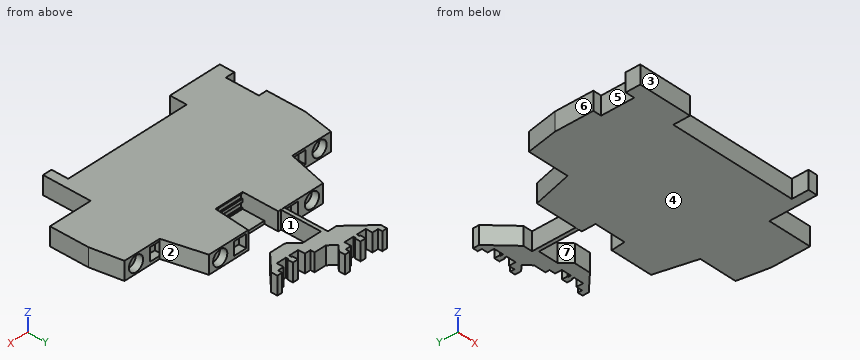
Autodesk Inventor part; units mm, degrees
ref_plane "1_1001_XY" through (7.05, 53.6, 2.5) normal (0, 1, 0) x (-1, 0, 0)
ref_plane "1_1001_YZ" through (7.05, 53.6, 2.5) normal (-1, 0, 0) x (0, 0, 1)
ref_plane "1_1001_ZX" through (7.05, 53.6, 2.5) normal (0, 0, 1) x (0, 1, 0)
sketch "Sketch_1" plane through (0, 0, 0) normal (0, 0, 1) x (1, 0, 0)
  line L0 (-32.2, -0.6) -> (-32.2, -4.6)
  line L1 (-32.2, -4.6) -> (-17.5, -4.6)
  line L2 (-17.5, -4.6) -> (-17.5, 0)
  line L3 (-17.5, 0) -> (17.5, 0)
  line L4 (17.5, 0) -> (17.5, -4.6)
  line L5 (17.5, -4.6) -> (20, -4.6)
  line L6 (20, -4.6) -> (20, 8.5)
  line L7 (20, 8.5) -> (32, 8.5)
  line L8 (32, 8.5) -> (32, 19.1)
  line L9 (32, 19.1) -> (30.5012, 27.6)
  line L10 (30.5012, 27.6) -> (-30.5012, 27.6)
  line L11 (-30.5012, 27.6) -> (-32, 19.1)
  line L12 (-32, 19.1) -> (-32, 8.5)
  line L13 (-32, 8.5) -> (-29.7, 8.5)
  line L14 (-29.7, 8.5) -> (-29.7, -0.6)
  line L15 (-29.7, -0.6) -> (-32.2, -0.6)
extrude "Extrusion1" add sketch "Sketch_1" along normal blind 5
sketch "Sketch_2" plane through (0, 0, 0) normal (0, 0, 1) x (1, 0, 0)
  line L0 (-19.1, 27.6) -> (-18.2, 27.6)
  line L1 (-18.2, 27.6) -> (-18.2, 15.1)
  line L2 (-18.2, 15.1) -> (19.2, 15.1)
  line L3 (19.2, 15.1) -> (19.2, 27.6)
  line L4 (19.2, 27.6) -> (20.1, 27.6)
  line L5 (20.1, 27.6) -> (17.3574, 38.6)
  line L6 (17.3574, 38.6) -> (5.7574, 38.6)
  line L7 (5.7574, 38.6) -> (4.9, 28.8)
  line L8 (4.9, 28.8) -> (-3.1, 28.8)
  line L9 (-3.1, 28.8) -> (-3.1, 38.6)
  line L10 (-3.1, 38.6) -> (-16.3574, 38.6)
  line L11 (-16.3574, 38.6) -> (-19.1, 27.6)
extrude "Extrusion2" add sketch "Sketch_2" along normal blind 5
sketch "Skizze_3" plane through (0, 0, 0) normal (0, 0, 1) x (1, 0, 0)
  line L0 (-3.1, 34.8) -> (-3.1, 28.8)
  line L1 (-3.1, 28.8) -> (5.9, 28.8)
  line L2 (5.9, 28.8) -> (5.9, 34.8)
  line L3 (5.9, 34.8) -> (-3.1, 34.8)
extrude "Extrusion3" add sketch "Skizze_3" along normal blind 0.8
sketch "Sketch_3" plane through (0.5, 0, 0) normal (1, 0, 0) x (0, 0, -1)
  line L0 (-4.7, 28.4) -> (-3.3, 28.4)
  line L1 (-3.3, 28.4) -> (-3.3, 28.8)
  line L2 (-3.3, 28.8) -> (-2.5, 28.8)
  line L3 (-2.5, 28.8) -> (-2.5, 28.4)
  line L4 (-2.5, 28.4) -> (-1.1, 28.4)
  line L5 (-1.1, 28.4) -> (-1.1, 29.8)
  line L6 (-1.1, 29.8) -> (-4.7, 29.8)
  line L7 (-4.7, 29.8) -> (-4.7, 28.4)
extrude "Extrusion4" cut sketch "Sketch_3" along normal mid plane 7.2
sketch "Sketch_4" plane through (0, 0, 2.5) normal (0, 0, 1) x (1, 0, 0)
  line L0 (27.1, 25.6) -> (27.1, 27.6)
  line L1 (27.1, 27.6) -> (29.2, 27.6)
  line L2 (29.2, 27.6) -> (29.2, 25.6)
  line L3 (29.2, 25.6) -> (27.1, 25.6)
  line L4 (27.1, 25.6) -> (27.1, 27.6)
revolve "Revolution1" cut sketch "Sketch_4" angle 360 about axis through (27.1, 25.6, 2.5) along (0, -1, 0)
sketch "Sketch_5" plane through (0, 0, 2.5) normal (0, 0, 1) x (1, 0, 0)
  line L0 (-27.1, 25.6) -> (-27.1, 27.6)
  line L1 (-27.1, 27.6) -> (-25, 27.6)
  line L2 (-25, 27.6) -> (-25, 25.6)
  line L3 (-25, 25.6) -> (-27.1, 25.6)
  line L4 (-27.1, 25.6) -> (-27.1, 27.6)
revolve "Revolution2" cut sketch "Sketch_5" angle 360 about axis through (-27.1, 25.6, 2.5) along (0, -1, 0)
sketch "Sketch_6" plane through (0, 0, 2.5) normal (0, 0, 1) x (1, 0, 0)
  line L0 (14.05, 36.6) -> (14.05, 38.6)
  line L1 (14.05, 38.6) -> (16.15, 38.6)
  line L2 (16.15, 38.6) -> (16.15, 36.6)
  line L3 (16.15, 36.6) -> (14.05, 36.6)
  line L4 (14.05, 36.6) -> (14.05, 38.6)
revolve "Revolution3" cut sketch "Sketch_6" angle 360 about axis through (14.05, 36.6, 2.5) along (0, -1, 0)
sketch "Sketch_7" plane through (0, 0, 2.5) normal (0, 0, 1) x (1, 0, 0)
  line L0 (-13.05, 36.6) -> (-13.05, 38.6)
  line L1 (-13.05, 38.6) -> (-10.95, 38.6)
  line L2 (-10.95, 38.6) -> (-10.95, 36.6)
  line L3 (-10.95, 36.6) -> (-13.05, 36.6)
  line L4 (-13.05, 36.6) -> (-13.05, 38.6)
revolve "Revolution4" cut sketch "Sketch_7" angle 360 about axis through (-13.05, 36.6, 2.5) along (0, -1, 0)
sketch "Skizze_15" plane through (0, 0, 2.5) normal (0, 0, 1) x (1, 0, 0)
  line L0 (-4.9, 36.6) -> (-3.9, 36.6)
  line L1 (-3.9, 36.6) -> (-3.9, 38.6)
  line L2 (-3.9, 38.6) -> (-4.9, 38.6)
  line L3 (-4.9, 38.6) -> (-4.9, 36.6)
extrude "Extrusion5" cut sketch "Skizze_15" along normal mid plane 4.1
sketch "Skizze_11" plane through (0, 0, 0.8) normal (0, 0, 1) x (1, 0, 0)
  line L0 (19.4, 25.6) -> (23, 25.6)
  line L1 (23, 25.6) -> (23, 27.6)
  line L2 (23, 27.6) -> (19.4, 27.6)
  line L3 (19.4, 27.6) -> (19.4, 25.6)
extrude "Extrusion6" cut sketch "Skizze_11" along normal blind 3.6
sketch "Skizze_12" plane through (0, 0, 0.8) normal (0, 0, 1) x (1, 0, 0)
  line L0 (-23, 25.6) -> (-19.4, 25.6)
  line L1 (-19.4, 25.6) -> (-19.4, 27.6)
  line L2 (-19.4, 27.6) -> (-23, 27.6)
  line L3 (-23, 27.6) -> (-23, 25.6)
extrude "Extrusion7" cut sketch "Skizze_12" along normal blind 3.6
sketch "Skizze_13" plane through (0, 0, 0.8) normal (0, 0, 1) x (1, 0, 0)
  line L0 (6.35, 36.6) -> (9.95, 36.6)
  line L1 (9.95, 36.6) -> (9.95, 38.6)
  line L2 (9.95, 38.6) -> (6.35, 38.6)
  line L3 (6.35, 38.6) -> (6.35, 36.6)
extrude "Extrusion8" cut sketch "Skizze_13" along normal blind 3.6
sketch "Skizze_14" plane through (0, 0, 0.8) normal (0, 0, 1) x (1, 0, 0)
  line L0 (-8.95, 36.6) -> (-5.35, 36.6)
  line L1 (-5.35, 36.6) -> (-5.35, 38.6)
  line L2 (-5.35, 38.6) -> (-8.95, 38.6)
  line L3 (-8.95, 38.6) -> (-8.95, 36.6)
extrude "Extrusion9" cut sketch "Skizze_14" along normal blind 3.6
sketch "Sketch_8" plane through (0, 0, 2.5) normal (0, 0, 1) x (1, 0, 0)
  line L0 (-13.75, 56.9029) -> (-7.4471, 50.6)
  line L1 (-7.4471, 50.6) -> (-4.9, 50.6)
  line L2 (-4.9, 50.6) -> (-4.9, 33.6)
  line L3 (-4.9, 33.6) -> (-3.9, 33.6)
  line L4 (-3.9, 33.6) -> (-3.9, 49.6)
  line L5 (-3.9, 49.6) -> (1.5103, 49.6)
  line L6 (1.5103, 49.6) -> (4.0103, 47.1)
  line L7 (4.0103, 47.1) -> (8.4471, 47.1)
  line L8 (8.4471, 47.1) -> (13.25, 51.9029)
  line L9 (13.25, 51.9029) -> (13.25, 53.6)
  line L10 (13.25, 53.6) -> (11.85, 53.6)
  line L11 (11.85, 53.6) -> (11.85, 52.45)
  line L12 (11.85, 52.45) -> (10.2, 52.45)
  line L13 (10.2, 52.45) -> (10.2, 50.6)
  line L14 (10.2, 50.6) -> (7.55, 50.6)
  line L15 (7.55, 50.6) -> (7.55, 51.3)
  line L16 (7.55, 51.3) -> (7.8, 51.3)
  line L17 (7.8, 51.3) -> (7.8, 52.8)
  line L18 (7.8, 52.8) -> (6.3, 52.8)
  line L19 (6.3, 52.8) -> (6.3, 51.3)
  line L20 (6.3, 51.3) -> (6.55, 51.3)
  line L21 (6.55, 51.3) -> (6.55, 50.6)
  line L22 (6.55, 50.6) -> (3.9, 50.6)
  line L23 (3.9, 50.6) -> (3.9, 52.45)
  line L24 (3.9, 52.45) -> (2.25, 52.45)
  line L25 (2.25, 52.45) -> (2.25, 53.6)
  line L26 (2.25, 53.6) -> (-1.0755, 53.6)
  line L27 (-1.0755, 53.6) -> (-2.8642, 55.3887)
  line L28 (-2.8642, 55.3887) -> (-1.35, 56.9029)
  line L29 (-1.35, 56.9029) -> (-1.35, 58.6)
  line L30 (-1.35, 58.6) -> (-2.75, 58.6)
  line L31 (-2.75, 58.6) -> (-2.75, 57.45)
  line L32 (-2.75, 57.45) -> (-4.4, 57.45)
  line L33 (-4.4, 57.45) -> (-4.4, 55.6)
  line L34 (-4.4, 55.6) -> (-7.05, 55.6)
  line L35 (-7.05, 55.6) -> (-7.05, 56.3)
  line L36 (-7.05, 56.3) -> (-6.8, 56.3)
  line L37 (-6.8, 56.3) -> (-6.8, 57.8)
  line L38 (-6.8, 57.8) -> (-8.3, 57.8)
  line L39 (-8.3, 57.8) -> (-8.3, 56.3)
  line L40 (-8.3, 56.3) -> (-8.05, 56.3)
  line L41 (-8.05, 56.3) -> (-8.05, 55.6)
  line L42 (-8.05, 55.6) -> (-10.7, 55.6)
  line L43 (-10.7, 55.6) -> (-10.7, 57.45)
  line L44 (-10.7, 57.45) -> (-12.35, 57.45)
  line L45 (-12.35, 57.45) -> (-12.35, 58.6)
  line L46 (-12.35, 58.6) -> (-13.75, 58.6)
  line L47 (-13.75, 58.6) -> (-13.75, 56.9029)
extrude "Extrusion10" add sketch "Sketch_8" along normal mid plane 4.95
ref_plane "1_1001_XY" through (7.05, 53.6, 2.5) normal (0, 1, 0) x (-1, 0, 0)
ref_plane "1_1001_YZ" through (7.05, 53.6, 2.5) normal (-1, 0, 0) x (0, 0, 1)
ref_plane "1_1001_ZX" through (7.05, 53.6, 2.5) normal (0, 0, 1) x (0, 1, 0)
ref_plane "1_1002_XY" through (-7.55, 58.6, 2.5) normal (0, 1, 0) x (-1, 0, 0)
ref_plane "1_1002_YZ" through (-7.55, 58.6, 2.5) normal (-1, 0, 0) x (0, 0, 1)
ref_plane "1_1002_ZX" through (-7.55, 58.6, 2.5) normal (0, 0, 1) x (0, 1, 0)
ref_plane "1_13_XY" through (0.4, 28.8, 2) normal (0, 1, 0) x (-1, 0, 0)
ref_plane "1_13_YZ" through (0.4, 28.8, 2) normal (-1, 0, 0) x (0, 0, 1)
ref_plane "1_13_ZX" through (0.4, 28.8, 2) normal (0, 0, 1) x (0, 1, 0)
ref_plane "1_14_XY" through (0.4, 28.8, 3.8) normal (0, 1, 0) x (-1, 0, 0)
ref_plane "1_14_YZ" through (0.4, 28.8, 3.8) normal (-1, 0, 0) x (0, 0, 1)
ref_plane "1_14_ZX" through (0.4, 28.8, 3.8) normal (0, 0, 1) x (0, 1, 0)
ref_plane "1_2_XY" through (-21.2, 27.6, 2.6) normal (0, 1, 0) x (1, 0, 0)
ref_plane "1_2_YZ" through (-21.2, 27.6, 2.6) normal (1, 0, 0) x (0, 0, -1)
ref_plane "1_2_ZX" through (-21.2, 27.6, 2.6) normal (0, 0, -1) x (0, 1, 0)
ref_plane "1_3_XY" through (-7.15, 38.6, 2.6) normal (0, 1, 0) x (1, 0, 0)
ref_plane "1_3_YZ" through (-7.15, 38.6, 2.6) normal (1, 0, 0) x (0, 0, -1)
ref_plane "1_3_ZX" through (-7.15, 38.6, 2.6) normal (0, 0, -1) x (0, 1, 0)
ref_plane "1_4_XY" through (8.15, 38.6, 2.6) normal (0, 1, 0) x (-1, 0, 0)
ref_plane "1_4_YZ" through (8.15, 38.6, 2.6) normal (-1, 0, 0) x (0, 0, 1)
ref_plane "1_4_ZX" through (8.15, 38.6, 2.6) normal (0, 0, 1) x (0, 1, 0)
ref_plane "1_5_XY" through (21.55, 27.6, 2.6) normal (0, 1, 0) x (-1, 0, 0)
ref_plane "1_5_YZ" through (21.55, 27.6, 2.6) normal (-1, 0, 0) x (0, 0, 1)
ref_plane "1_5_ZX" through (21.55, 27.6, 2.6) normal (0, 0, 1) x (0, 1, 0)
ref_plane "1_6_XY" through (-27.1, 27.6, 2.5) normal (0, 1, 0) x (1, 0, 0)
ref_plane "1_6_YZ" through (-27.1, 27.6, 2.5) normal (1, 0, 0) x (0, 0, -1)
ref_plane "1_6_ZX" through (-27.1, 27.6, 2.5) normal (0, 0, -1) x (0, 1, 0)
ref_plane "1_7_XY" through (-13.05, 38.6, 2.5) normal (0, 1, 0) x (1, 0, 0)
ref_plane "1_7_YZ" through (-13.05, 38.6, 2.5) normal (1, 0, 0) x (0, 0, -1)
ref_plane "1_7_ZX" through (-13.05, 38.6, 2.5) normal (0, 0, -1) x (0, 1, 0)
ref_plane "1_8_XY" through (14.05, 38.6, 2.5) normal (0, 1, 0) x (-1, 0, 0)
ref_plane "1_8_YZ" through (14.05, 38.6, 2.5) normal (-1, 0, 0) x (0, 0, 1)
ref_plane "1_8_ZX" through (14.05, 38.6, 2.5) normal (0, 0, 1) x (0, 1, 0)
ref_plane "1_9_XY" through (27.1, 27.6, 2.5) normal (0, 1, 0) x (-1, 0, 0)
ref_plane "1_9_YZ" through (27.1, 27.6, 2.5) normal (-1, 0, 0) x (0, 0, 1)
ref_plane "1_9_ZX" through (27.1, 27.6, 2.5) normal (0, 0, 1) x (0, 1, 0)
ref_plane "MD_XY" through (0, 0, 0) normal (0, -1, 0) x (0, 0, 1)
ref_plane "MD_YZ" through (0, 0, 0) normal (0, 0, 1) x (-1, 0, 0)
ref_plane "MD_ZX" through (0, 0, 0) normal (-1, 0, 0) x (0, -1, 0)
ref_plane "OP_XY" through (-32.2, -4.6, 0) normal (0, 1, 0) x (0, 0, 1)
ref_plane "OP_YZ" through (-32.2, -4.6, 0) normal (0, 0, 1) x (1, 0, 0)
ref_plane "OP_ZX" through (-32.2, -4.6, 0) normal (1, 0, 0) x (0, 1, 0)
ref_plane "a1_XY" through (27.1, 12.6, 2.5) normal (0, 1, 0) x (-1, 0, 0)
ref_plane "a1_YZ" through (27.1, 12.6, 2.5) normal (-1, 0, 0) x (0, 0, 1)
ref_plane "a1_ZX" through (27.1, 12.6, 2.5) normal (0, 0, 1) x (0, 1, 0)
ref_plane "a2_XY" through (14.05, 23.6, 2.5) normal (0, 1, 0) x (-1, 0, 0)
ref_plane "a2_YZ" through (14.05, 23.6, 2.5) normal (-1, 0, 0) x (0, 0, 1)
ref_plane "a2_ZX" through (14.05, 23.6, 2.5) normal (0, 0, 1) x (0, 1, 0)
ref_plane "b3_XY" through (-13.05, 23.6, 2.5) normal (0, 1, 0) x (1, 0, 0)
ref_plane "b3_YZ" through (-13.05, 23.6, 2.5) normal (1, 0, 0) x (0, 0, -1)
ref_plane "b3_ZX" through (-13.05, 23.6, 2.5) normal (0, 0, -1) x (0, 1, 0)
ref_plane "b4_XY" through (-27.1, 12.6, 2.5) normal (0, 1, 0) x (1, 0, 0)
ref_plane "b4_YZ" through (-27.1, 12.6, 2.5) normal (1, 0, 0) x (0, 0, -1)
ref_plane "b4_ZX" through (-27.1, 12.6, 2.5) normal (0, 0, -1) x (0, 1, 0)
ref_plane "j5_XY" through (0.4, 22.8, 2) normal (0, 1, 0) x (-1, 0, 0)
ref_plane "j5_YZ" through (0.4, 22.8, 2) normal (-1, 0, 0) x (0, 0, 1)
ref_plane "j5_ZX" through (0.4, 22.8, 2) normal (0, 0, 1) x (0, 1, 0)
ref_plane "j6_XY" through (0.4, 22.8, 3.8) normal (0, 1, 0) x (-1, 0, 0)
ref_plane "j6_YZ" through (0.4, 22.8, 3.8) normal (-1, 0, 0) x (0, 0, 1)
ref_plane "j6_ZX" through (0.4, 22.8, 3.8) normal (0, 0, 1) x (0, 1, 0)
ref_plane "m7_XY" through (7.05, 53.6, 2.5) normal (0, 1, 0) x (-1, 0, 0)
ref_plane "m7_YZ" through (7.05, 53.6, 2.5) normal (-1, 0, 0) x (0, 0, 1)
ref_plane "m7_ZX" through (7.05, 53.6, 2.5) normal (0, 0, 1) x (0, 1, 0)
ref_plane "m8_XY" through (-7.55, 58.6, 2.5) normal (0, 1, 0) x (-1, 0, 0)
ref_plane "m8_YZ" through (-7.55, 58.6, 2.5) normal (-1, 0, 0) x (0, 0, 1)
ref_plane "m8_ZX" through (-7.55, 58.6, 2.5) normal (0, 0, 1) x (0, 1, 0)
ref_plane "z10_XY" through (8.15, 38.6, 2.6) normal (0, 1, 0) x (-1, 0, 0)
ref_plane "z10_YZ" through (8.15, 38.6, 2.6) normal (-1, 0, 0) x (0, 0, 1)
ref_plane "z10_ZX" through (8.15, 38.6, 2.6) normal (0, 0, 1) x (0, 1, 0)
ref_plane "z11_XY" through (-7.15, 38.6, 2.6) normal (0, 1, 0) x (1, 0, 0)
ref_plane "z11_YZ" through (-7.15, 38.6, 2.6) normal (1, 0, 0) x (0, 0, -1)
ref_plane "z11_ZX" through (-7.15, 38.6, 2.6) normal (0, 0, -1) x (0, 1, 0)
ref_plane "z12_XY" through (-21.2, 27.6, 2.6) normal (0, 1, 0) x (1, 0, 0)
ref_plane "z12_YZ" through (-21.2, 27.6, 2.6) normal (1, 0, 0) x (0, 0, -1)
ref_plane "z12_ZX" through (-21.2, 27.6, 2.6) normal (0, 0, -1) x (0, 1, 0)
ref_plane "z9_XY" through (21.55, 27.6, 2.6) normal (0, 1, 0) x (-1, 0, 0)
ref_plane "z9_YZ" through (21.55, 27.6, 2.6) normal (-1, 0, 0) x (0, 0, 1)
ref_plane "z9_ZX" through (21.55, 27.6, 2.6) normal (0, 0, 1) x (0, 1, 0)
sketch "Sketch15" plane through (-27.1, 25.6, 2.5) normal (0, 1, 0) x (1, 0, 0)
  circle A0 centre (0, 0) radius 2.1
sketch "Sketch16" plane through (-13.05, 36.6, 2.5) normal (0, 1, 0) x (1, 0, 0)
  circle A0 centre (0, 0) radius 2.1
sketch "Sketch17" plane through (14.05, 36.6, 2.5) normal (0, 1, 0) x (1, 0, 0)
  circle A0 centre (0, 0) radius 2.1
sketch "Sketch18" plane through (27.1, 25.6, 2.5) normal (0, 1, 0) x (1, 0, 0)
  circle A0 centre (0, 0) radius 2.1
properties part number "280-519_LO"
The model under review builds one solid part; all positions refer to its coordinate system, in mm. Face numbers are marked on the shaded views. A direction names the side the tool comes from. Coordinates: 2 decimals unless noted, no trailing zeros. Write each loop counter-clockwise with the first axis right and the second up, starting at its lowest first coordinate (ties: lowest second). Pieces come first, ordered by that corner, then holes. Notation, with made-up numbers: (82, 8.25) - (130, 8.25) arc R21 cw to (130, 33.25) - close; hole circle Ø2 at (38.5, 27). An arc over 180 degrees is marked (long way). Answer in a Markdown table with one row per item. Add a question column.
Q1. Draft analysis for pull direction Y (two halves, no side actions). For the marked faces 1, 2, 3 and 4, state which applies: +Y half, -Y half, draft (parallel to the pull), parting line (faces both ways), or undercut.
Q2. Consider section A-A on x = -27.1. Give the boundary of the cut face in (y, z).
Q3. Consider section D-D on x = 14.05. Give the boundary of the cut face in (y, z), then the cut area to 3 significant figures.
Q4. Clearance check with flat-ended pins moving along their axes: pin 1 (1.5 mm diameter, centred on x = 1, y = 12, fed in from -Z); pin 2 (0.6 mm diameter, centred on y = 52, z = 1.5, fed in from +X); pin 3 (0.6 mm diameter, centred on y = 56, z = 1.5, fed in from +X); pin 4 (0.6 mm diameter, centred on y = 37.5, z = 2.5, fed in from +X). State where each tip first meets the part, or that it passes through.
Q5. To check wall thickness, follow line 1 along Y through (x, z) = (-0.5, 1.9); line 2 along Y through (x, z) = (4.5, 4.45); line 3 along X through (y, z) = (17, 4.65). State the ranges of each line that lie inside material, in increasing order. Write a range as from..to.
Q6. Consider section C-C on y = 4. Give the boundary of the cut face in (x, z), then the cut area to 4 significant figures.
Q7. For the marked faces 5, 6 and 7, list the 3-axis set-ups (+Z, -Z, +X, -X, +Y, -Y) from which the entire face can be reached by the end or side of a thin tool; tool diameter is ignored.
Q8. Consider section B-B on x = 3. Give the boundary of the cut face in (y, z) (3 decimals), then the cut area to 3 significant figures.
Answers below:
| question | item | result |
|---|---|---|
| 1 | face 1 | undercut |
| 1 | face 2 | +Y half |
| 1 | face 3 | -Y half |
| 1 | face 4 | draft |
| 2 | outline | (-4.6, 0) - (27.6, 0) - (27.6, 0.4) - (25.6, 0.4) - (25.6, 4.6) - (27.6, 4.6) - (27.6, 5) - (-4.6, 5) - close |
| 3 | outline | (0, 0) - (38.6, 0) - (38.6, 0.4) - (36.6, 0.4) - (36.6, 4.6) - (38.6, 4.6) - (38.6, 5) - (0, 5) - close |
| 3 | area | 185 mm² |
| 4 | pin 1 | z = 0 |
| 4 | pin 2 | x = 13.25 |
| 4 | pin 3 | x = -1.95 |
| 4 | pin 4 | x = 17.71 |
| 5 | line 1 | 0..28.4, 49.6..53.6 |
| 5 | line 2 | 0..28.8, 47.1..50.6 |
| 5 | line 3 | -32..32 |
| 6 | outline | (-29.7, 0) - (20, 0) - (20, 5) - (-29.7, 5) - close |
| 6 | area | 248.5 mm² |
| 7 | face 5 | +Z, -Z, -X |
| 7 | face 6 | +Z, -Z, -X, +Y |
| 7 | face 7 | +Z, -Z |
| 8 | outline | (0, 0) - (34.8, 0) - (34.8, 0.8) - (28.8, 0.8) - (28.8, 1.1) - (28.4, 1.1) - (28.4, 2.5) - (28.8, 2.5) - (28.8, 3.3) - (28.4, 3.3) - (28.4, 4.7) - (28.8, 4.7) - (28.8, 5) - (0, 5) - close; (48.11, 0.025) - (52.45, 0.025) - (52.45, 4.975) - (48.11, 4.975) - close |
| 8 | area | 169 mm² |
